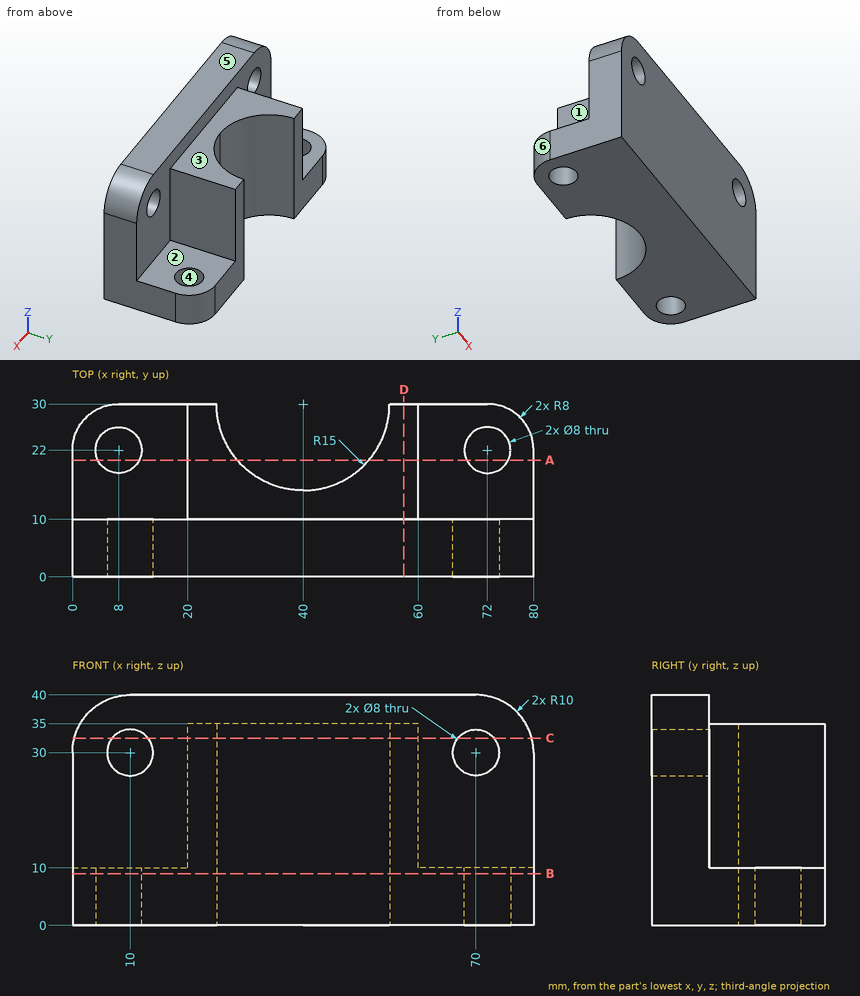
Can you work these out from the drawing? Everything is in mm from the part's minimum corner. A direction names the side the tool comes from. Give positions to 0.01 mm unless a question says otherwise; leave off trailing zeros. Order: outer loops, then holes, each group sorted by start corner. A loop starts at its lowest first (then second) coordinate and runs counter-clockwise, first axis right, second up.
Item 1: I need wall thicknesses on line 1 (X direction, y = 4, z = 30); line 2 (Z direction, x = 10, y = 7.5); line 3 (Y direction, x = 8, z = 6.5). Which ranges of each line are inside material? Lowest first, please.
Item 2: If we section it at C-C, the plane z = 32.5: Write out the boundary of the cut face in (x, y).
Item 3: If we section it at D-D, the plane x = 57.5: Write out the boundary of the cut face in (y, z), plus the area to 3 significant figures.
Item 4: I'm going to push flat-ended pins straight in: pin 1 (6 mm diameter, centred on y = 23.5, z = 18, fed in from +X); pin 2 (9 mm diameter, centred on x = 8, y = 22, fed in from +Z); pin 3 (9 mm diameter, centred on x = 70, z = 30, fed in from +Y). Where does each tip first touch, or does it pass through?
Item 5: If we mould it in two halves opening along Y, with no side actions, what happens to the marked faces 4, 5 and 6? For each: pulls with the +Y half, pulls with the -Y half, needs draft (parallel to the pull), parting line crosses it, or undercut.
Item 6: If we section it at B-B, the plane z = 9: Write out the boundary of the cut face in (x, y).
Item 7: For the marked faces 1, 2 and 3, which set-ups out of +Z, -Z, +X, -X, +Y, -Y let a thin tool reach every point of the face, with its end or its side?
Item 8: If we section it at A-A, the plane y = 20.25: Write out the boundary of the cut face in (x, z).
Values:
1. line 1: x = 0 to 6, 14 to 66, 74 to 80
1. line 2: z = 0 to 26, 34 to 40
1. line 3: y = 0 to 18, 26 to 30
2. outline: (0.32, 0) - (6.88, 0) - (6.88, 10) - (0.32, 10) - close; (13.12, 0) - (66.88, 0) - (66.88, 10) - (60, 10) - (60, 30) - (55, 30) arc R15 cw to (25, 30) - (20, 30) - (20, 10) - (13.12, 10) - close; (73.12, 0) - (79.68, 0) - (79.68, 10) - (73.12, 10) - close
3. outline: (0, 0) - (30, 0) - (30, 35) - (10, 35) - (10, 40) - (0, 40) - close
3. area: 1,100 mm2
4. pin 1: stops at x = 60
4. pin 2: stops at z = 10
4. pin 3: stops at y = 10
5. face 4: undercut
5. face 5: needs draft
5. face 6: pulls with the +Y half
6. outline: (0, 0) - (80, 0) - (80, 22) arc R8 ccw to (72, 30) - (55, 30) arc R15 cw to (25, 30) - (8, 30) arc R8 ccw to (0, 22) - close; hole circle Ø8 at (8, 22); hole circle Ø8 at (72, 22)
7. face 1: +Z, -X, +Y
7. face 2: +Z, +X, +Y
7. face 3: +Z, +X, -X, +Y
8. outline: (0, 0) - (4.4, 0) - (4.4, 10) - (0, 10) - close; (11.6, 0) - (28.6, 0) - (28.6, 35) - (20, 35) - (20, 10) - (11.6, 10) - close; (51.4, 0) - (68.4, 0) - (68.4, 10) - (60, 10) - (60, 35) - (51.4, 35) - close; (75.6, 0) - (80, 0) - (80, 10) - (75.6, 10) - close
